Check sheet for the modelled part. Datum: model origin and axes. Units: mm. A direction names the side the tool comes from. Round coordinates to 2 decimals unless told otherwise and drop trailing zeros. Order: outer loops, then holes, each group sorted by start corner. A loop starts at its lowest first (then second) coordinate and runs counter-clockwise, first axis right, second up.
(1) Mould release check, pull along Z, two halves, no side actions. Record for faces 4 (the conical face through (7.41, 23.52, 69.84)), 5 (the flat face through (4, -46, 4)), 6 (the cylindrical face through (-26.36, -5.85, 51.02)), 7 (the conical face through (-20.61, -0.61, -49.88)): released by +Z, released by -Z, zero draft, split by the parting line, or undercut.
(2) Tool access check on faces 1 (the cylindrical face through (0, -46, 22)), 2 (the cylindrical face through (6.56, -3.65, -28.24)), 3 (the flat face through (10.7, 5, -37)). Record the directions out of +Z, -Z, +X, -X, +Y, -Y that give a thin tool (end or side, any length) a straight path to the whole face; none if there is none.
(3) Thickness scan on probe 1 along Y at (x, z) = (5, -33); probe 2 along Y at (x, z) = (8, -33); probe 3 along Z at (x, y) = (-30, -31). Record the ranges inside material, lowest first.
(4) Sectioned sample at A-A, the plane z = 60. Enter the section's corners in (x, y).
(5) Depth check by flat-ended pin: pin 1 (6 mm diameter, centred on y = 12.5, z = 54.5, fed in from -X); pin 2 (12 mm diameter, centred on x = -26.5, y = 38, fed in from +Z); pin 3 (6.5 mm diameter, centred on x = 0, z = 0.5, fed in from -Y); pin 4 (5 mm diameter, centred on y = -29, z = -21.5, fed in from -X). Enter the tip coordinate at first touch or a pass-through.
```python
from build123d import *

# Parameters (mm, degrees)
CHAMFER1_SIZE      = 2.5
CUT_EXTRUDE1_DEPTH = 5.5
SKETCH5_W          = 36
SKETCH5_H          = 43
CUT_EXTRUDE2_DEPTH = 12.3
SKETCH6_R          = 6
CUT_EXTRUDE3_DEPTH = 8.4
SKETCH7_R          = 6
FILLET2_R          = 2


with BuildPart() as part:
    # Sketch1 → Revolve1 (revolve)
    with BuildSketch(Plane(origin=(0, 0, 0), x_dir=(0, 0, -1), z_dir=(1, 0, 0))):
        Polygon((-70, 0), (-70, 27), (-35, 27), (-35, 22), (-30, 22), (-30, 49), (18, 49), (18, 23), (50, 23), (50, 0), align=None)
    revolve(axis=Axis((0, 0, 127.018539307), (0, 0, -1)))

    # Chamfer1
    chamfer1_edges = [part.edges().sort_by_distance(p)[0] for p in [
        (0, -27, 70),
        (0, -23, -50),
        (0, -49, 30),
    ]]
    chamfer(chamfer1_edges, length=CHAMFER1_SIZE)

    # Sketch3 → Cut-Extrude1 (cut)
    with BuildSketch(Plane(origin=(0, -49, 0), x_dir=(-1, 0, 0), z_dir=(0, -1, 0))):
        with BuildLine():
            Line((-4, -18), (-4, 10))
            ThreePointArc((-4, 10), (0, 14), (4, 10))
            Line((4, 10), (4, -18))
            ThreePointArc((4, -18), (0, -22), (-4, -18))
        make_face()
    extrude(amount=-CUT_EXTRUDE1_DEPTH, mode=Mode.SUBTRACT)

    # Sketch5 → Cut-Extrude2 (cut)
    with BuildSketch(Plane(origin=(10.7, 0, 0), x_dir=(0, 0, -1), z_dir=(1, 0, 0))):
        with Locations((36, 1.5)):
            Rectangle(SKETCH5_W, SKETCH5_H)
    extrude(amount=CUT_EXTRUDE2_DEPTH, mode=Mode.SUBTRACT)

    # Sketch6 → Cut-Extrude3 (cut)
    with BuildSketch(Plane(origin=(10.7, 0, 0), x_dir=(0, 0, -1), z_dir=(1, 0, 0))):
        with Locations((33, 0)):
            Circle(SKETCH6_R)
    extrude(amount=-CUT_EXTRUDE3_DEPTH, mode=Mode.SUBTRACT)

    # Sketch7 → Cut-Loft1 section 0
    with BuildSketch(Plane(origin=(2.3, 0, 0), x_dir=(0, 0, -1), z_dir=(1, 0, 0)), mode=Mode.PRIVATE) as cut_loft1_s0:
        with Locations((33, 0)):
            Circle(SKETCH7_R)
    loft([Vertex(0, 0, -33), cut_loft1_s0.sketch], mode=Mode.SUBTRACT)

    # Fillet2
    fillet2_edges = [part.edges().sort_by_distance(p)[0] for p in [
        (0, -22, 30),
        (0, -22, 35),
    ]]
    fillet(fillet2_edges, radius=FILLET2_R)


solid = part.part
```
Derived:
1. face 4: released by +Z
1. face 5: undercut
1. face 6: zero draft
1. face 7: released by -Z
2. face 1: -Y
2. face 2: +X
2. face 3: -Z, +X, +Y
3. probe 1: y = -22.45 to -6, 6 to 22.45
3. probe 2: y = -21.56 to -6, 6 to 21.56
3. probe 3: z = -18 to 30
4. outline: circle Ø54 at (0, 0)
5. pin 1: stops at x = -25.27
5. pin 2: stops at z = 30
5. pin 3: stops at y = -43.5
5. pin 4: passes through
